Check sheet for the modelled part. Datum: model origin and axes. Units: mm. Face numbers are marked on the shaded views. A direction names the side the tool comes from. Give positions to 0.01 mm unless a question says otherwise; leave off trailing zeros. Loops run counter-clockwise (first coordinate to the right, second up) from the corner with the lowest first, then second, coordinate; pieces in that order, holes last. Notation, with made-up numbers: M -22.75,87 L 23.25,87 A27 cw 23.25,116 Z; hole C 2.5,85 d7. An arc over 180 degrees is marked long. Put each result on its own line as item: value. Start each with the question number.
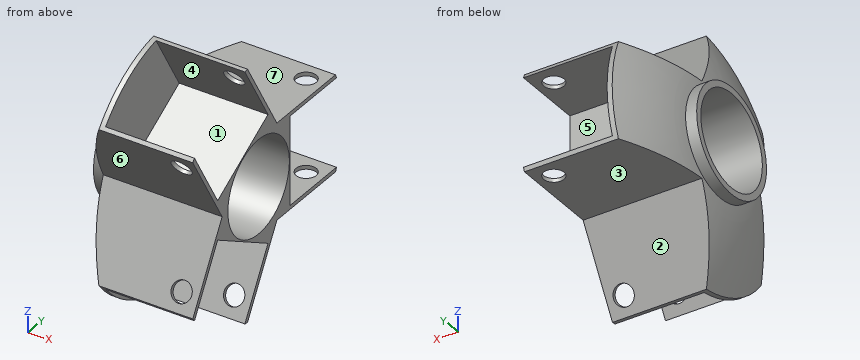
Autodesk Inventor part; units mm, degrees
ref_plane "YZ Plane" through (0, 0, 0) normal (1, 0, 0) x (0, 1, 0)
ref_plane "XZ Plane" through (0, 0, 0) normal (0, 1, 0) x (-1, 0, 0)
ref_plane "XY Plane" through (0, 0, 0) normal (0, 0, 1) x (1, 0, 0)
sketch "Boceto1" plane through (0, 0, 0) normal (0, 1, 0) x (-1, 0, 0)
  line L0 (116.8368, 0) -> (-138.9188, 0) construction
  line L1 (0, 201.6217) -> (0, -202.3506) construction
  line L2 (-16.9655, 0) -> (-16.9655, 50)
  line L3 (-16.9655, 50) -> (20.0345, 50)
  spline S0 degree 2 poles (20.0345, 50) (29.4829, 31.811) (30.3202, 17.0589) knots 0 0 0 1 1 1
  line L4 (30.3202, 17.0589) -> (30.3202, 0)
  line L5 (30.3202, 0) -> (-16.9655, 0)
  point P0 (0, 0)
  point P1 (27.7444, 31.3016)
  dimension "d0" = 50
  dimension "d1" = 37
  dimension "d2" = 30.3202
  dimension "d3" = 47.2856
  dimension "d4" = 86.5167
  dimension "d5" = 32.9412
  dimension "d6" = 2.5758
  dimension "d7" = 18.6984
  dimension "d8" = 151.6217
  dimension "d9" = 252.3506
  dimension "d10" = 169.239
revolve "Revolución1" add sketch "Boceto1" angle 360 about axis through (-116.8368, 0, 0) along (1, 0, 0)
sketch "Boceto2" plane through (-30.3202, 0, 0) normal (-1, 0, 0) x (0, 0, 1)
  circle A0 centre (0, 0) radius 17.0589
  circle A1 centre (0, 0) radius 21
  point P0 (17.0589, 0)
  dimension "d12" = 42
extrude "Extrusión1" add sketch "Boceto2" along normal mid plane 8 contours A0 | A1
sketch "Boceto3" plane through (-34.3202, 0, 0) normal (-1, 0, 0) x (0, 0, 1)
  circle A0 centre (0, 0) radius 18.5
  dimension "d15" = 37
extrude "Extrusión2" cut sketch "Boceto3" against normal blind 60
sketch "Boceto4" plane through (-34.3202, 0, 0) normal (-1, 0, 0) x (0, 0, 1)
  circle A0 centre (0, 0) radius 50
  line L0 (-19, 46.2493) -> (-19, 8.9443)
  circle A1 centre (0, 0) radius 21
  line L1 (19, 46.2493) -> (19, 8.9443)
  line L2 (0, 54.3807) -> (0, -24.3097) construction
  line L3 (-65.0318, 0) -> (77.048, 0) construction
  circle A2 centre (0, 0) radius 50 construction
  circle A3 centre (0, 0) radius 21 construction
  line L4 (-30.5531, -39.5791) -> (1.754, -20.9266)
  line L5 (-49.5531, -6.6702) -> (-17.246, 11.9823)
  circle A4 centre (0, 0) radius 21 construction
  circle A5 centre (0, 0) radius 50 construction
  line L6 (49.5531, -6.6702) -> (17.246, 11.9823)
  line L7 (30.5531, -39.5791) -> (-1.754, -20.9266)
  circle A6 centre (0, 0) radius 21 construction
  circle A7 centre (0, 0) radius 50 construction
  point P0 (19, 10.9697)
  point P1 (-19, 10.9697)
  point P2 (0, -21.9393)
  dimension "d18" = 38
  dimension "d21" = 360
extrude "Extrusión3" cut sketch "Boceto4" against normal blind 60 contours A0 L6 L1 | L0 L5 A0 | A0 L4 L7
sketch "Boceto5" plane through (-29.8214, -21.9393, 0) normal (0, -0.866, -0.5) x (1, 0, 0)
  line L0 (0, 35.9798) -> (0, -55.1659) construction
  line L1 (-10.6314, 0) -> (61.9402, 0) construction
  circle A0 centre (40, 28) radius 4
  point P0 (29.8214, -10.9697)
  point P1 (0, 0)
  dimension "d25" = 40
  dimension "d26" = 28
  dimension "d27" = 8
extrude "Extrusión4" cut sketch "Boceto5" against normal blind 60
pattern_circular "Patrón circular1" count 3 over 360 about axis through (-34.3202, 0, 0) along (1, 0, 0) of "Extrusión4"
sketch "Boceto6" plane through (16.9655, 10.9697, 19) normal (1, 0, 0) x (0, 0, -1)
  line L0 (36.5, 8.0303) -> (1.5, 8.0303)
  line L1 (1.5, 8.0303) -> (1.5, 43.8507)
  line L2 (1.5, 43.8507) -> (36.5, 43.8507)
  line L3 (36.5, 43.8507) -> (36.5, 8.0303)
  line L4 (19, 66.8345) -> (19, -59.037) construction
  line L5 (-55.9645, -10.9697) -> (107.3868, -10.9697) construction
  line L6 (-19.7258, -53.5353) -> (-37.2258, -23.2244)
  line L7 (11.2955, -35.6251) -> (-19.7258, -53.5353)
  line L8 (-37.2258, -23.2244) -> (-6.2045, -5.3142)
  line L9 (-6.2045, -5.3142) -> (11.2955, -35.6251)
  line L10 (75.2258, -23.2244) -> (57.7258, -53.5353)
  line L11 (44.2045, -5.3142) -> (75.2258, -23.2244)
  line L12 (57.7258, -53.5353) -> (26.7045, -35.6251)
  line L13 (26.7045, -35.6251) -> (44.2045, -5.3142)
  point P0 (19, -10.9697)
  point P1 (25.7111, -10.9697)
  dimension "d33" = 35
  dimension "d34" = 35.8203
  dimension "d35" = 19
  dimension "d38" = 360
extrude "Extrusión5" cut sketch "Boceto6" against normal blind 35
Q1. Access from +Z, -Z, +X, -X, +Y, -Y to the whole of each face (thin tool, end or side, straight path). Record for the marked faces 4, 5, 6 and 7.
Q2. Thickness scan on line 1 along Y through (x, z) = (0, -15); line 2 along Z through (x, y) = (-4, 24.5); line 3 along Y through (x, z) = (9.5, -13). Record the ranges inside material, lowest first. Write a range as [from, to].
Q3. Mould release check, pull along Y, two halves, no side actions. Record for the marked faces 1, 2 and 3: pulls with the +Y half, pulls with the -Y half, needs draft (parallel to the pull), parting line crosses it, or undercut.
Q4. Section check A-A, the plane x = -7. Record the cut outline in (y, z).
Q5. Section check B-B, the plane x = 11.5. Give the number of separate pieces and of enclosed holes in the cut face, then the cut area to 3 significant figures.
Q6. Depth check by flat-ended pin: P1, Ø12, axis at x = 5, y = 10.5, coming from the +Z side; P2, Ø21, axis at y = -12, z = -25, coming from the +X side; P3, Ø22.5, axis at x = 1.5, y = 40, coming from the +Z side; P4, Ø22.5, axis at x = -0.5, y = 28, coming from the -Z side. Enter the tip coordinate at first touch or a pass-through.
Found:
1. face 4: +X
1. face 5: +X, +Y
1. face 6: +X, -X, -Y
1. face 7: +Z, +X, -X, +Y
2. line 1: y = [-30.6, -28.87], [-12.02, -10.83], [10.83, 19]
2. line 2: z = [-19, -17.5], [17.5, 19]
2. line 3: y = [-29.44, -27.71], [-15.48, -13.16], [13.16, 19]
3. face 1: undercut
3. face 2: pulls with the +Y half
3. face 3: needs draft
4. outline: M -39.58,-30.55 A50 ccw -38.57,-31.81 L -24.66,-7.7 L 5.66,-25.2 L -8.26,-49.31 A50 ccw -6.67,-49.55 L 10.97,-19 L 46.25,-19 A50 ccw 46.84,-17.5 L 19,-17.5 L 19,17.5 L 46.84,17.5 A50 ccw 46.25,19 L 10.97,19 L -6.67,49.55 A50 ccw -8.26,49.31 L 5.66,25.2 L -24.66,7.7 L -38.57,31.81 A50 ccw -39.58,30.55 L -21.94,0 Z; hole C 0,0 d37
5. separate pieces: 7
5. enclosed holes: 1
5. area: 645 mm^2
6. P1: stops at z = 30.21
6. P2: stops at x = 16.97
6. P3: stops at z = 19
6. P4: stops at z = -19
